```python
from build123d import *

# Parameters (mm, degrees)
EXTRUDE_1_DEPTH     = 7.8
SKETCH_3_R          = 1.5
CUT_EXTRUDE_1_DEPTH = 12
SKETCH_9_R          = 1.5
CUT_EXTRUDE_2_DEPTH = 12
SKETCH_10_R         = 1.5
CUT_EXTRUDE_3_DEPTH = 12
CUT_EXTRUDE_4_DEPTH = 8.8
SKETCH_14_W         = 50.2
SKETCH_14_H         = 10
EXTRUDE_2_DEPTH     = 3


with BuildPart() as part:
    # 草圖1 → 填料-伸長1 (new body)
    with BuildSketch(Plane.XY):
        Polygon((-25, 70), (25, 70), (73.121778265, -13.349364905), (48.121778265, -56.650635095), (-48.121778265, -56.650635095), (-73.121778265, -13.349364905), align=None)
    extrude(amount=EXTRUDE_1_DEPTH)

    # 草圖3 → 除料-伸長1 (cut)
    with BuildSketch(Plane(origin=(-49.060889132, 28.325317547, 0), x_dir=(0, 0, 1), z_dir=(-0.866025404, 0.5, 0))):
        with Locations((3.9, 40.2)):
            Circle(SKETCH_3_R)
        with Locations((3.9, 30)):
            Circle(SKETCH_3_R)
        with Locations((3.9, -30)):
            Circle(SKETCH_3_R)
        with Locations((3.9, -40.2)):
            Circle(SKETCH_3_R)
    extrude(amount=-CUT_EXTRUDE_1_DEPTH, mode=Mode.SUBTRACT)

    # 草圖9 → 除料-伸長2 (cut)
    with BuildSketch(Plane.XZ.offset(56.650635095)):
        with Locations((-30, 3.9)):
            Circle(SKETCH_9_R)
        with Locations((-40.2, 3.9)):
            Circle(SKETCH_9_R)
        with Locations((40.2, 3.9)):
            Circle(SKETCH_9_R)
        with Locations((30, 3.9)):
            Circle(SKETCH_9_R)
    extrude(amount=-CUT_EXTRUDE_2_DEPTH, mode=Mode.SUBTRACT)

    # 草圖10 → 除料-伸長3 (cut)
    with BuildSketch(Plane(origin=(49.060889132, 28.325317547, 0), x_dir=(0, 0, -1), z_dir=(0.866025404, 0.5, 0))):
        with Locations((-3.9, 40.2)):
            Circle(SKETCH_10_R)
        with Locations((-3.9, 30)):
            Circle(SKETCH_10_R)
        with Locations((-3.9, -30)):
            Circle(SKETCH_10_R)
        with Locations((-3.9, -40.2)):
            Circle(SKETCH_10_R)
    extrude(amount=-CUT_EXTRUDE_3_DEPTH, mode=Mode.SUBTRACT)

    # 草圖13 → 除料-伸長4 (cut, through all)
    with BuildSketch(Plane.XY.offset(7.8)):
        Polygon((-61.574772881, -13.349364905), (-19.226497308, 60), (19.226497308, 60), (61.574772881, -13.349364905), (42.348275573, -46.650635095), (-42.348275573, -46.650635095), align=None)
    extrude(amount=-CUT_EXTRUDE_4_DEPTH, mode=Mode.SUBTRACT)

    # 草圖14 → 填料-伸長2 (add)
    with BuildSketch(Plane.XY.offset(7.8)):
        Polygon((-27.850635095, 45.062555182), (-36.510889132, 50.062555182), (-61.610889132, 6.588079912), (-52.950635095, 1.588079912), align=None)
        Polygon((36.510889132, 50.062555182), (27.850635095, 45.062555182), (52.950635095, 1.588079912), (61.610889132, 6.588079912), align=None)
        with Locations((0, -51.650635095)):
            Rectangle(SKETCH_14_W, SKETCH_14_H)
    extrude(amount=EXTRUDE_2_DEPTH)


solid = part.part
```
Can you work these out from the model? Positions are in its coordinate system, mm. A direction names the side the tool comes from. Coordinates: 2 decimals unless noted, no trailing zeros. Loops run counter-clockwise (first coordinate to the right, second up) from the corner with the lowest first, then second, coordinate; pieces in that order, holes last. Notation, with made-up numbers: (41.25, 3) - (52.25, 3) arc R25 cw to (52.25, 33) - close; hole circle Ø4 at (-33, 87). An arc over 180 degrees is marked (long way). Use a Markdown table: item, result.
Item 1: I want a section at B-B on x = 23. Give the number of separate pieces and of enclosed holes in the cut face, and give its area (3 significant figures).
Numbers:
| item | result |
|---|---|
| separate pieces | 2 |
| enclosed holes | 1 |
| area | 229 mm2 |
Item 2: I want a section at C-C on y = -24.5. Please give me the cut outline in (x, z), and give its area (3 significant figures).
Numbers:
| item | result |
|---|---|
| outline | (-66.68, 0) - (-55.14, 0) - (-55.14, 7.8) - (-66.68, 7.8) - close; (55.14, 0) - (66.68, 0) - (66.68, 7.8) - (55.14, 7.8) - close |
| area | 180 mm2 |
Item 3: For faces 1 (the face through (53, -30, 7.8)), 2 (the face through (25.1, -52, 9)), 3 (the face through (52.096, -29.767, 3.955)), 4 (the face through (-31.5, -51.72, 3.97)), which set-ups out of +Z, -Z, +X, -X, +Y, -Y let a thin tool reach every point of the face, with its end or its side?
Numbers:
| item | result |
|---|---|
| face 1 | +Z, +X, -Y |
| face 2 | +Z, +X, +Y, -Y |
| face 3 | +Z, -Z |
| face 4 | -Y |
Item 4: If I drill on probe 1 along Z at (x, y) = (-40.2, -50.5); probe 2 along Y at (x, z) = (-8.5, 5.25); probe 3 along X at (y, z) = (2, 1.5), over which ranges is the centre line in solid material (lowest first)? Write a range as from..to.
Numbers:
| item | result |
|---|---|
| probe 1 | z = 0..2.4, 5.4..7.8 |
| probe 2 | y = -56.65..-46.65, 60..70 |
| probe 3 | x = -64.26..-52.71, 52.71..64.26 |
Item 5: I want a section at A-A on y = 30. Please give me the cut outline in (x, z), and give its area (3 significant figures).
Numbers:
| item | result |
|---|---|
| outline | (-48.09, 0) - (-36.55, 0) - (-36.55, 10.8) - (-48.09, 10.8) - close; (36.55, 0) - (48.09, 0) - (48.09, 10.8) - (36.55, 10.8) - close |
| area | 249 mm2 |
Item 6: Will these pins go through, and if not, where does the flat tip stop? pin 1 (12.5 mm diameter, centred on x = 1, y = 60.5, fed in from +Z); pin 2 (12 mm diameter, centred on x = 42.5, y = 51, fed in from -Z); pin 3 (2 mm diameter, centred on x = 50, z = 8, fed in from -Y); pin 4 (3.5 mm diameter, centred on x = 40.2, z = 3.9, fed in from +Y).
Numbers:
| item | result |
|---|---|
| pin 1 | stops at z = 7.8 |
| pin 2 | stops at z = 0 |
| pin 3 | stops at y = -55.09 |
| pin 4 | stops at y = 46.7 |
Item 7: We'd pull the mould along Z, two halves only. Please class faces 5 (the face through (-54, -30, 7.8)), 6 (the face through (32.241, 47.598, 9.279)), 7 (the face through (59.05, 1.17, 4.1)): released by +Z, released by -Z, zero draft, split by the parting line, or undercut.
Numbers:
| item | result |
|---|---|
| face 5 | released by +Z |
| face 6 | zero draft |
| face 7 | undercut |
